from build123d import *

# Parameters (mm, degrees)
SKETCH1_W           = 23
SKETCH1_H           = 23
BOSS_EXTRUDE1_DEPTH = 11
SKETCH2_W           = 17
SKETCH2_H           = 17
CUT_EXTRUDE1_DEPTH  = 7.5
SKETCH3_W           = 18
SKETCH3_H           = 19
BOSS_EXTRUDE2_DEPTH = 14
SKETCH4_R           = 1
CUT_EXTRUDE2_DEPTH  = 23


with BuildPart() as part:
    # Sketch1 → Boss-Extrude1 (new body)
    with BuildSketch(Plane(origin=(0, 0, 0), x_dir=(1, 0, 0), z_dir=(0, 1, 0))):
        with Locations((10.331746032, -10.598253968)):
            Rectangle(SKETCH1_W, SKETCH1_H)
    extrude(amount=-BOSS_EXTRUDE1_DEPTH)

    # Sketch2 → Cut-Extrude1 (cut)
    with BuildSketch(Plane(origin=(0, 0, 0), x_dir=(1, 0, 0), z_dir=(0, 1, 0))):
        with Locations((10.331746032, -10.598253968)):
            Rectangle(SKETCH2_W, SKETCH2_H)
    extrude(amount=-CUT_EXTRUDE1_DEPTH, mode=Mode.SUBTRACT)

    # Sketch3 → Boss-Extrude2 (add)
    with BuildSketch(Plane.XZ.offset(11)):
        with Locations((10.331746032, 8.598253968)):
            Rectangle(SKETCH3_W, SKETCH3_H)
    extrude(amount=BOSS_EXTRUDE2_DEPTH)

    # Sketch4 → Cut-Extrude2 (cut)
    with BuildSketch(Plane.ZY.offset(1.168253968)):
        with Locations((8.598253968, -2.006935825)):
            Circle(SKETCH4_R)
        with Locations((16.598253968, -2.006935825)):
            Circle(SKETCH4_R)
    extrude(amount=-CUT_EXTRUDE2_DEPTH, mode=Mode.SUBTRACT)


solid = part.part
Could you check a few things on this model? Use its own coordinates, in mm. A direction names the side the tool comes from. Round coordinates to 2 decimals unless told otherwise and drop trailing zeros. Order: outer loops, then holes, each group sorted by start corner. A loop starts at its lowest first (then second) coordinate and runs counter-clockwise, first axis right, second up. Notation, with made-up numbers: M -18,44 L -7,44 A26 cw -7,66 Z; hole C 51,-38 d8. An arc over 180 degrees is marked long. One line per item, written item: value.
(1) Which directions (+Z, -Z, +X, -X, +Y, -Y) give clear straight access to the entire face, cutting with the end or side of a thin tool? Please do faces 1 (the flat face through (10, -7.5, 10)), 2 (the flat face through (10, -25, 9)), 3 (the flat face through (1.332, -18, 8)), 4 (the flat face through (10, -18, 18.098)).
Ans:
face 1: +Y
face 2: +Z, -Z, +X, -X, -Y
face 3: +Z, -Z, -X, -Y
face 4: +Z, +X, -X, -Y
(2) I'm going to push flat-ended pins straight in: P1, Ø4, axis at y = -17.5, z = 12, coming from the +X side; P2, Ø7, axis at x = 11, y = -17, coming from the +Z side; P3, Ø1.2, axis at y = -2.01, z = 8.6, coming from the -X side; P4, Ø7, axis at y = -16, z = 8, coming from the -X side. Where does each tip first touch, or does it pass through?
Ans:
P1: stops at x = 19.33
P2: stops at z = 18.1
P3: passes through
P4: stops at x = 1.33
(3) Imagine slicing it at A-A (y = -5.25). Write out the boundary of the cut face in (x, z), and give its area (3 significant figures).
Ans:
outline: M -1.17,-0.9 L 21.83,-0.9 L 21.83,22.1 L -1.17,22.1 Z; hole M 1.83,2.1 L 18.83,2.1 L 18.83,19.1 L 1.83,19.1 Z
area: 240 mm^2
(4) If we mould it in two halves opening along X, with no side actions, what happens to faces 5 (the flat face through (19.332, -18, 8)), 6 (the flat face through (18.832, -4, 11)), 7 (the cylindrical face through (0.31, -2.39, 17.52))? For each: released by +X, released by -X, zero draft, split by the parting line, or undercut.
Ans:
face 5: released by +X
face 6: undercut
face 7: zero draft
(5) Imagine slicing it at D-D (z = 16.5). Write out the boundary of the cut face in (x, y).
Ans:
outline: M -1.17,-11 L 1.33,-11 L 1.33,-25 L 19.33,-25 L 19.33,-11 L 21.83,-11 L 21.83,-3 L 18.83,-3 L 18.83,-7.5 L 1.83,-7.5 L 1.83,-3 L -1.17,-3 Z; M -1.17,-1.01 L 1.83,-1.01 L 1.83,0 L -1.17,0 Z; M 18.83,-1.01 L 21.83,-1.01 L 21.83,0 L 18.83,0 Z
(6) Imagine slicing it at C-C (x = 17.5). Write out the boundary of the cut face in (y, z).
Ans:
outline: M -25,-0.9 L 0,-0.9 L 0,2.1 L -7.5,2.1 L -7.5,19.1 L 0,19.1 L 0,22.1 L -11,22.1 L -11,18.1 L -25,18.1 Z
(7) I need wall thicknesses on line 1 along X through (y, z) = (-5.5, 12); line 2 along Z through (x, y) = (7.5, -1.75); line 3 along Y through (x, z) = (19.5, 11.25). Which ranges of each line are inside material? Lowest first, please. Write a range as from..to.
Ans:
line 1: x = -1.17..1.83, 18.83..21.83
line 2: z = -0.9..2.1, 19.1..22.1
line 3: y = -11..0
(8) Imagine slicing it at B-B (z = 6.5). Write out the boundary of the cut face in (x, y), and give its area (4 significant figures).
Ans:
outline: M -1.17,-11 L 1.33,-11 L 1.33,-25 L 19.33,-25 L 19.33,-11 L 21.83,-11 L 21.83,0 L 18.83,0 L 18.83,-7.5 L 1.83,-7.5 L 1.83,0 L -1.17,0 Z
area: 377.5 mm^2
